CAD build for the part. Positions are in the model's coordinates, mm. Face numbers are marked on the shaded views. A direction names the side the tool comes from. Round coordinates to 2 decimals unless told otherwise and drop trailing zeros. Order: outer loops, then holes, each group sorted by start corner. A loop starts at its lowest first (then second) coordinate and runs counter-clockwise, first axis right, second up. Notation, with made-up numbers: (79.25, 22.25) -> (108.25, 22.25) arc R11 cw to (108.25, 37.25) -> close; hole circle Ø10 at (-30, -33). An arc over 180 degrees is marked (long way). Return JSON: item names as keys, results as strings. Group by question number.
Q1. Cut at A-A (y = 5.75). Count the separate pieces of the cut face and the enclosed holes in it, then the cut area to 3 significant figures.
Q2. Which spindle directions (+Z, -Z, +X, -X, +Y, -Y) get a long thin tool onto all of the face, cutting with end or side? Do the marked faces 4 and 5. Say none if no direction does.
Q3. Cut at B-B (z = 2). Write the cut outline in (x, y) (3 decimals), then the cut area to 3 significant figures.
Q4. Flat gauge pins, fed straight in: pin 1 (12 mm diameter, centred on x = -10.5, z = -25, fed in from -Y); pin 2 (12 mm diameter, centred on y = 14, z = -27.5, fed in from -X); pin 3 (2.5 mm diameter, centred on x = -21.43, z = -41.75, fed in from -Y). Where does each tip first touch, or does it go through?
Q5. Mould opens along Z. For the marked faces 1, 2 and 3 say: +Z half, -Z half, draft (parallel to the pull), parting line (faces both ways), or undercut.
Q6. Probe line 1 along Z through (x, y) = (-8.5, 11); line 2 along X through (y, z) = (10.25, -42); line 3 along X through (y, z) = (17, -34.5). List the from-to ranges inside material, lowest first.
Autodesk Inventor part; units mm, degrees
ref_plane "YZ Plane" through (0, 0, 0) normal (1, 0, 0) x (0, 1, 0)
ref_plane "XZ Plane" through (0, 0, 0) normal (0, 1, 0) x (-1, 0, 0)
ref_plane "XY Plane" through (0, 0, 0) normal (0, 0, 1) x (1, 0, 0)
sketch "Sketch1" plane through (0, 0, 0) normal (0, 1, 0) x (-1, 0, 0)
  line L0 (-18.5654, 9.2536) -> (2.9346, 9.2536)
  line L1 (2.9346, 9.2536) -> (2.9346, -17.7464)
  line L2 (2.9346, -17.7464) -> (-18.5654, -17.7464)
  line L3 (-18.5654, -17.7464) -> (-18.5654, 9.2536)
  circle A0 centre (-15.5654, 6.2536) radius 0.875
  line L4 (-17.5654, 3.454) -> (-17.5654, -16.6136)
  line L5 (2.9346, 8.2536) -> (-13.3293, 8.2536)
  line L6 (-17.5654, 3.454) -> (-17.5654, 4.0175)
  line L7 (-17.5654, -16.6136) -> (-17.5654, -17.7464)
  arc A1 (-17.5654, 4.0175) -> (-13.3293, 8.2536) centre (-15.5654, 6.2536) ccw
  point P0 (0, 0)
  dimension "d0" = 21.5
  dimension "d2" = 27
  dimension "d3" = 3
  dimension "d4" = 3
  dimension "d6" = 1.75
  dimension "d7" = 1
  dimension "d8" = 1
extrude "Extrusion1" add sketch "Sketch1" along normal blind 20 contours L0 L1 L5 A1 L6 L4 L7 L2 L3
sketch "Sketch2" plane through (0, 0, 0) normal (0, -1, 0) x (1, 0, 0)
  line L0 (18.5654, 9.2536) -> (-2.9346, 9.2536)
  line L1 (-2.9346, 9.2536) -> (-2.9346, -17.7464)
  line L2 (-2.9346, -17.7464) -> (18.5654, -17.7464)
  line L3 (18.5654, -17.7464) -> (18.5654, 9.2536)
  point P0 (0, 0)
extrude "Extrusion2" add sketch "Sketch2" along normal blind 1
mirror "Mirror1" about plane through (18.5654, 0, -17.7464) normal (0, 0, -1) of "Extrusion1", "Extrusion2"
mirror "Mirror2" about plane through (-2.9346, 0, 8.2536) normal (-1, 0, 0) of "Extrusion1", "Extrusion2", "Mirror1"
sketch "Sketch3" plane through (18.5654, -1, 9.2536) normal (0, 0, 1) x (1, 0, 0)
  line L0 (0, 0) -> (-43, 0)
  arc A0 (-43, 0) -> (0, 0) centre (-21.5, 230.625) ccw
  line L1 (-40.8006, -1) -> (-1.6118, -1)
  point P0 (-18.5654, 1)
  dimension "d13" = 1
extrude "Extrusion3" add sketch "Sketch3" against normal blind 54
fillet "Fillet1" radius 2 8 edges at (-24.4346, -1, -17.7464) (-2.9346, -2, -44.7464) (-24.4346, 9.5, -44.7464) (18.5654, 9.5, -44.7464) (-24.4346, 9.5, 9.2536) (-2.9346, -2, 9.2536) (18.5654, 9.5, 9.2536) (18.5654, -1, -17.7464)
sketch "Sketch4" plane through (0, 0, 0) normal (0, 1, 0) x (1, 0, 0)
  line L0 (-38.0807, 38.7464) -> (-17.4346, 38.7464)
  line L1 (-17.4346, 38.7464) -> (-17.4346, -3.2536)
  line L2 (-17.4346, -3.2536) -> (-38.0807, -3.2536)
  line L3 (-38.0807, -3.2536) -> (-38.0807, 38.7464)
  line L4 (-24.4346, 42.7464) -> (-24.4346, -7.2536)
  arc A0 (-23.4346, 39.5104) -> (-19.1985, 43.7464) centre (-21.4346, 41.7464) ccw
  arc A1 (-19.1985, -8.2536) -> (-23.4346, -4.0175) centre (-21.4346, -6.2536) ccw
  point P0 (0, 0)
  dimension "d17" = 7
extrude "Extrusion4" cut sketch "Sketch4" along normal mid plane 50
properties part number "cuerpo"
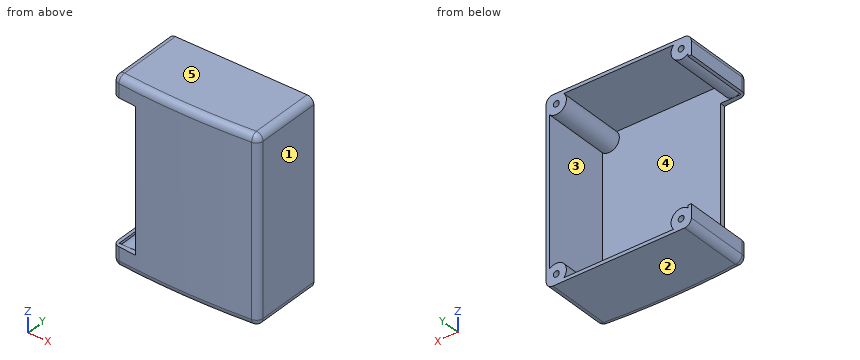
Solution:
{
 "1": {"separate pieces": "1", "enclosed holes": "4", "area": "223 mm²"},
 "2": {"face 4": "+Y", "face 5": "+Z, +X, -X, +Y, -Y"},
 "3": {"outline": "(-17.435, -1.546) arc R231.625 ccw to (16.735, -1.163) arc R2 ccw to (18.565, 0.829) -> (18.565, 20) -> (17.565, 20) -> (17.565, 0) -> (-17.435, 0) -> close", "area": "81.9 mm²"},
 "4": {"pin 1": "stops at y = -1.99", "pin 2": "stops at x = 17.57", "pin 3": "stops at y = -1.36"},
 "5": {"face 1": "draft", "face 2": "-Z half", "face 3": "undercut"},
 "6": {"line 1": "z = -44.75 to -43.75, 8.25 to 9.25", "line 2": "x = -24.43 to -22.27, -20.6 to -18.45, 12.58 to 14.73, 16.4 to 18.57", "line 3": "x = 17.57 to 18.57"}
}
